Could you check a few things on this model? Use its own coordinates, in mm. Face numbers are marked on the shaded views. Round coordinates to 2 decimals unless told otherwise and drop trailing zeros.
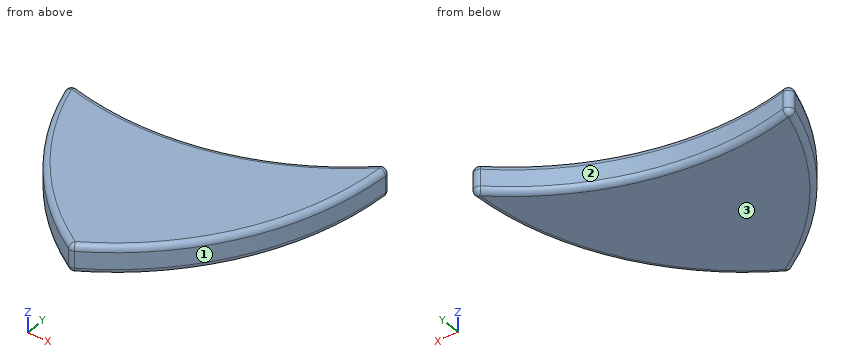
```python
from build123d import *

# Parameters (mm, degrees)
ESTRUSIONE_ESTRUSIONE1_DEPTH = 5
RACCORDO1_R                  = 1


with BuildPart() as part:
    # Schizzo1 → Estrusione-Estrusione1 (new body)
    with BuildSketch(Plane.XY):
        with BuildLine():
            ThreePointArc((-48.296291314, -12.940952255), (-39.667667015, -30.43807145), (-25, -43.301270189))
            ThreePointArc((-25, -43.301270189), (-6.698729811, -25), (0, 0))
            ThreePointArc((0, 0), (-22.414386804, -12.940952255), (-48.296291314, -12.940952255))
        make_face()
    extrude(amount=ESTRUSIONE_ESTRUSIONE1_DEPTH)

    # Raccordo1
    raccordo1_edges = [part.edges().sort_by_distance(p)[0] for p in [
        (-39.667667015, -30.43807145, 5),
        (-39.667667015, -30.43807145, 0),
        (-22.414386804, -12.940952255, 0),
        (-6.698729811, -25, 0),
        (-6.698729811, -25, 5),
        (-25, -43.301270189, 2.5),
        (-48.296291314, -12.940952255, 2.5),
        (0, 0, 2.5),
        (-22.414386804, -12.940952255, 5),
    ]]
    fillet(raccordo1_edges, radius=RACCORDO1_R)


solid = part.part
```
Q1. If I drill on L1, parallel to Y at x = -41.5, z = 1; L2, parallel to X at y = -24, z = 3; L3, parallel to Y at x = -25, z = 3.05, over which ranges is the centre line in solid material (lowest first)?
Q2. I'm going to push a flat-ended pin straight in: pin 1 Ø1.5 at (y, z) = (-25.5, 2.5) entering from -X. Where does the tip first touch, or does it pass through?
Q3. We'd pull the mould along X, two halves only. Please class the marked faces 1, 2 and 3: pulls with the +X half, pulls with the -X half, needs draft (parallel to the pull), parting line crosses it, or undercut.
Results found:
1. L1: y = -27.89 to -14.27
1. L2: x = -43.86 to -6.14
1. L3: y = -43.14 to -13.56
2. pin 1: stops at x = -43.44
3. face 1: pulls with the +X half
3. face 2: undercut
3. face 3: needs draft
